```python
from build123d import *

# Parameters (mm, degrees)
EXTRUDE_1_DEPTH            = 10
EXTRUDE_START              = -100
EXTRUDE_3_DEPTH            = 80
SKETCH_5_W                 = 80
SKETCH_5_H                 = 60
CUT_EXTRUDE_2_DEPTH        = 110
FILLET_1_R                 = 50
FILLET_2_R                 = 200
SKETCH_7_R                 = 9
CUT_EXTRUDE_6_DEPTH        = 6
SKETCH_10_R                = 6
CUT_EXTRUDE_7_DEPTH        = 28
SKETCH_12_R                = 15
EXTRUDE_5_DEPTH            = 4
SKETCH_13_R                = 9
CUT_EXTRUDE_9_DEPTH        = 4
CUT_EXTRUDE_START          = -2.25
SKETCH_14_R                = 9.75
CUT_EXTRUDE_4141_DEPTH     = 1
CHAMFER_1_SIZE             = 1
CHAMFER_1_OF_MIRROR_1_SIZE = 1
SKETCH_16_R                = 13
CUT_EXTRUDE_10_DEPTH       = 0.75
CUT_EXTRUDE_START_2        = -0.75
SKETCH_17_R                = 13
CUT_EXTRUDE_11_DEPTH       = 0.75
CHAMFER_2_SIZE             = 30
CHAMFER_2_SIZE2            = 60
CHAMFER_3_SIZE             = 60
CHAMFER_3_SIZE2            = 30
FILLET_3_R                 = 10


with BuildPart() as part:
    # 草图1 → 凸台-拉伸1 (new body)
    with BuildSketch(Plane(origin=(0, 0, 0), x_dir=(1, 0, 0), z_dir=(0, 1, 0))):
        Polygon((-100, 0), (100, 0), (100, 180), (50, 300), (-50, 300), (-100, 180), align=None)
    extrude(amount=EXTRUDE_1_DEPTH)

    # 草图4 → 凸台-拉伸3 (add)
    with BuildSketch(Plane.XY.offset(EXTRUDE_START)):
        with BuildLine():
            Line((0, 29), (0, 10))
            Line((0, 10), (30, 10))
            Line((30, 10), (30, 40))
            ThreePointArc((30, 40), (21.213203436, 61.213203436), (0, 70))
            Line((0, 70), (0, 51))
            ThreePointArc((0, 51), (7.778174593, 47.778174593), (11, 40))
            ThreePointArc((11, 40), (7.778174593, 32.221825407), (0, 29))
        make_face()
        with BuildLine():
            Line((-30, 10), (0, 10))
            Line((0, 10), (0, 29))
            ThreePointArc((0, 29), (-11, 40), (0, 51))
            Line((0, 51), (0, 70))
            ThreePointArc((0, 70), (-21.213203436, 61.213203436), (-30, 40))
            Line((-30, 40), (-30, 10))
        make_face()
    extrude(amount=-EXTRUDE_3_DEPTH)

    # 草图5 → 切除-拉伸2 (cut)
    with BuildSketch(Plane(origin=(0, 10, 0), x_dir=(1, 0, 0), z_dir=(0, 1, 0))):
        with Locations((0, 140)):
            Rectangle(SKETCH_5_W, SKETCH_5_H)
    extrude(amount=CUT_EXTRUDE_2_DEPTH, mode=Mode.SUBTRACT)

    # 圆角1
    fillet_1_edges = [part.edges().sort_by_distance(p)[0] for p in [
        (-50, 5, -300),
        (50, 5, -300),
    ]]
    fillet(fillet_1_edges, radius=FILLET_1_R)

    # 圆角2
    fillet_2_edges = [part.edges().sort_by_distance(p)[0] for p in [
        (-100, 5, -180),
        (100, 5, -180),
    ]]
    fillet(fillet_2_edges, radius=FILLET_2_R)

    # 草图7 → 切除-拉伸6 (cut)
    with BuildSketch(Plane(origin=(0, 10, 0), x_dir=(1, 0, 0), z_dir=(0, 1, 0))):
        with Locations(Location((45, 30, 0), (0, 0, 270))):
            Circle(SKETCH_7_R)
    cut_extrude_6 = extrude(amount=-CUT_EXTRUDE_6_DEPTH, mode=Mode.SUBTRACT)

    # 草图10 → 切除-拉伸7 (cut)
    with BuildSketch(Plane(origin=(0, 4, 0), x_dir=(1, 0, 0), z_dir=(0, 1, 0))):
        with Locations(Location((45, 30, 0), (0, 0, 270))):
            Circle(SKETCH_10_R)
    cut_extrude_7 = extrude(amount=-CUT_EXTRUDE_7_DEPTH, mode=Mode.SUBTRACT)

    # 草图12 → 凸台-拉伸5 (add)
    with BuildSketch(Plane(origin=(0, 10, 0), x_dir=(1, 0, 0), z_dir=(0, 1, 0))):
        with Locations(Location((45, 30, 0), (0, 0, 270))):
            Circle(SKETCH_12_R)
    extrude_5 = extrude(amount=EXTRUDE_5_DEPTH)

    # 草图13 → 切除-拉伸9 (cut)
    with BuildSketch(Plane(origin=(0, 14, 0), x_dir=(1, 0, 0), z_dir=(0, 1, 0))):
        with Locations(Location((45, 30, 0), (0, 0, 270))):
            Circle(SKETCH_13_R)
    cut_extrude_9 = extrude(amount=-CUT_EXTRUDE_9_DEPTH, mode=Mode.SUBTRACT)

    # 草图14 → Cut-Extrude 4141 (cut)
    with BuildSketch(Plane(origin=(0, 14, 0), x_dir=(1, 0, 0), z_dir=(0, 1, 0)).offset(CUT_EXTRUDE_START)):
        with Locations(Location((45, 30, 0), (0, 0, 270))):
            Circle(SKETCH_14_R)
    cut_extrude_4141 = extrude(amount=-CUT_EXTRUDE_4141_DEPTH, mode=Mode.SUBTRACT)

    # 倒角1
    chamfer_1_edges = [part.edges().sort_by_distance(p)[0] for p in [
        (45, 14, -45),
        (45, 14, -39),
    ]]
    chamfer(chamfer_1_edges, length=CHAMFER_1_SIZE)

    # 镜向1: 切除-拉伸6, 切除-拉伸7, 凸台-拉伸5, 切除-拉伸9, Cut-Extrude 4141 across plane
    add(cut_extrude_6.mirror(Plane.ZY), mode=Mode.SUBTRACT)
    add(cut_extrude_7.mirror(Plane.ZY), mode=Mode.SUBTRACT)
    add(extrude_5.mirror(Plane.ZY))
    add(cut_extrude_9.mirror(Plane.ZY), mode=Mode.SUBTRACT)
    add(cut_extrude_4141.mirror(Plane.ZY), mode=Mode.SUBTRACT)

    # 倒角1 of 镜向1
    chamfer_1_of_mirror_1_edges = [part.edges().sort_by_distance(p)[0] for p in [
        (-45, 14, -45),
        (-45, 14, -39),
    ]]
    chamfer(chamfer_1_of_mirror_1_edges, length=CHAMFER_1_OF_MIRROR_1_SIZE)

    # 草图16 → 切除-拉伸10 (cut)
    with BuildSketch(Plane.XY.offset(-100)):
        with Locations((0, 40)):
            Circle(SKETCH_16_R)
    extrude(amount=-CUT_EXTRUDE_10_DEPTH, mode=Mode.SUBTRACT)

    # 草图17 → 切除-拉伸11 (cut)
    with BuildSketch(Plane(origin=(0, 0, -180), x_dir=(-1, 0, 0), z_dir=(0, 0, -1)).offset(CUT_EXTRUDE_START_2)):
        with Locations(Location((0, 40, 0), (0, 0, 180))):
            Circle(SKETCH_17_R)
    extrude(amount=CUT_EXTRUDE_11_DEPTH, mode=Mode.SUBTRACT)

    # 倒角2
    chamfer_2_edges = [part.edges().sort_by_distance(p)[0] for p in [
        (100, 5, 0),
    ]]
    chamfer_2_side = [part.faces().sort_by_distance(p)[0] for p in [
        (0, 5, 0),
    ]]
    chamfer(chamfer_2_edges, length=CHAMFER_2_SIZE, length2=CHAMFER_2_SIZE2, reference=chamfer_2_side[0])

    # 倒角3
    chamfer_3_edges = [part.edges().sort_by_distance(p)[0] for p in [
        (-100, 5, 0),
    ]]
    chamfer_3_side = [part.faces().sort_by_distance(p)[0] for p in [
        (-100, 5, -70),
    ]]
    chamfer(chamfer_3_edges, length=CHAMFER_3_SIZE, length2=CHAMFER_3_SIZE2, reference=chamfer_3_side[0])

    # 圆角3
    fillet_3_edges = [part.edges().sort_by_distance(p)[0] for p in [
        (100, 5, -60),
        (70, 5, 0),
        (-70, 5, 0),
        (-100, 5, -60),
    ]]
    fillet(fillet_3_edges, radius=FILLET_3_R)


solid = part.part
```
Part model, mm, in its own coordinate system. A direction names the side the tool comes from. Round coordinates to 2 decimals unless told otherwise and drop trailing zeros. Loops run counter-clockwise (first coordinate to the right, second up) from the corner with the lowest first, then second, coordinate; pieces in that order, holes last.
Item 1: Cut at D-D, the plane z = -30. State how many separate pieces and enclosed holes the cut face has, then the cut area to 3 significant figures.
Item 2: Cut at C-C, the plane y = 62. Give the cut face in (x, z), then the cut area to 3 significant figures.
Item 3: 3-axis set-ups, long thin cutter, end or side, ignore diameter. For faces 5 (the face through (6, 27, -180)), 6 (the face through (6, 27, -100)), 7 (the face through (39.07, 11.26, -37.74)), 8 (the face through (-1.69, 27.11, -179.62)): which of +Z, -Z, +X, -X, +Y, -Y reach the whole face in a straight line?
Item 4: Mould opens along Z. For faces 1 (the face through (-55, 14, -33)), 2 (the face through (-69.011, 5.07, -1.453)), 3 (the face through (-39.07, 11.26, -37.74)), 4 (the face through (73.87, 4.93, -242.71)) say: +Z half, -Z half, draft (parallel to the pull), parting line (faces both ways), or undercut.
Item 5: Cut at B-B, the plane x = 45. Give the cut face in (y, z).
Item 6: Drill centre lines: line 1 (X direction, y = 12, z = -30); line 2 (X direction, y = 11, z = -30); line 3 (Z direction, x = -20, y = 12). Where is each one in solid material? Low to high.
Item 7: Cut at A-A, the plane y = 36.5. Give the cut face in (x, z), then the cut area to 3 significant figures.
Item 8: Drop flat-ended pins along their axis: P1, Ø18, axis at x = -10, y = 47.5, coming from the -Z side; P2, Ø14.5, axis at x = 44.5, z = -26.5, coming from the +Y side; P3, Ø3, axis at y = 27, z = -105.5, coming from the +X side; P4, Ø8, axis at x = 2, y = 37, coming from the +Z side. Give the stop position or say it passes through.
A:
1. separate pieces: 3
1. enclosed holes: 0
1. area: 1,480 mm2
2. outline: (-20.4, -180) - (20.4, -180) - (20.4, -170) - (-20.4, -170) - close; (-20.4, -110) - (20.4, -110) - (20.4, -100) - (-20.4, -100) - close
2. area: 816 mm2
3. face 5: -Z, +X, -X, +Y
3. face 6: +Z, +X, -X, +Y
3. face 7: none
3. face 8: -Z
4. face 1: draft
4. face 2: +Z half
4. face 3: undercut
4. face 4: -Z half
5. outline: (0, -291.2) - (10, -291.2) - (10, -45) - (13, -45) - (14, -44) - (14, -40) - (13, -39) - (11.75, -39) - (11.75, -39.75) - (10.75, -39.75) - (10.75, -39) - (4, -39) - (4, -36) - (0, -36) - close; (0, -24) - (4, -24) - (4, -21) - (10.75, -21) - (10.75, -20.25) - (11.75, -20.25) - (11.75, -21) - (13, -21) - (14, -20) - (14, -16) - (13, -15) - (10, -15) - (10, 0) - (0, 0) - close
6. line 1: x = -60 to -54, -36 to -30, 30 to 36, 54 to 60
6. line 2: x = -60 to -54.75, -35.25 to -30, 30 to 35.25, 54.75 to 60
6. line 3: z = -180 to -170, -110 to -100
7. outline: (-30, -180) - (-12.52, -180) - (-12.52, -179.25) - (-10.43, -179.25) - (-10.43, -170) - (-30, -170) - close; (-30, -110) - (-10.43, -110) - (-10.43, -100.75) - (-12.52, -100.75) - (-12.52, -100) - (-30, -100) - close; (10.43, -179.25) - (12.52, -179.25) - (12.52, -180) - (30, -180) - (30, -170) - (10.43, -170) - close; (10.43, -110) - (30, -110) - (30, -100) - (12.52, -100) - (12.52, -100.75) - (10.43, -100.75) - close
7. area: 777 mm2
8. P1: stops at z = -180
8. P2: stops at y = 14
8. P3: stops at x = 30
8. P4: passes through
